```python
from build123d import *

# Parameters (mm, degrees)
EXTRUDE_1_DEPTH     = 5
FILLET_1_R          = 2
SKETCH_2_R          = 1.5
CUT_EXTRUDE_1_DEPTH = 26.495097568
SKETCH_6_R          = 1.5
CUT_EXTRUDE_2_DEPTH = 37.400549446


with BuildPart() as part:
    # 草图1 → 凸台-拉伸1 (new body)
    with BuildSketch(Plane.XY):
        Polygon((9, 20), (9, 12), (-9, 12), (-9, 20), (-15, 20), (-15, -20), (-9, -20), (-9, -12), (9, -12), (9, -20), (15, -20), (15, 20), align=None)
    extrude(amount=EXTRUDE_1_DEPTH)

    # 圆角1
    fillet_1_edges = [part.edges().sort_by_distance(p)[0] for p in [
        (9, -20, 2.5),
        (9, -12, 2.5),
        (-9, -12, 2.5),
        (-9, -20, 2.5),
        (-9, 20, 2.5),
        (-9, 12, 2.5),
        (9, 12, 2.5),
        (9, 20, 2.5),
    ]]
    fillet(fillet_1_edges, radius=FILLET_1_R)

    # 草图2 → 切除-拉伸1 (cut, through all)
    with BuildSketch(Plane.XY.offset(5)):
        with Locations((-5, 5)):
            Circle(SKETCH_2_R)
        with Locations(Location((5, -5, 0), (0, 0, 180))):
            Circle(SKETCH_2_R)
    extrude(amount=-CUT_EXTRUDE_1_DEPTH, mode=Mode.SUBTRACT)

    # 草图6 → 切除-拉伸2 (cut, through all)
    with BuildSketch(Plane(origin=(15, 0, 0), x_dir=(0, 0, -1), z_dir=(1, 0, 0))):
        with Locations(Location((-2.5, 16, 0), (0, 0, 90))):
            Circle(SKETCH_6_R)
        with Locations(Location((-2.5, -16, 0), (0, 0, 90))):
            Circle(SKETCH_6_R)
    extrude(amount=-CUT_EXTRUDE_2_DEPTH, mode=Mode.SUBTRACT)


solid = part.part
```
Here's how the part is built. I have some questions about the finished solid (model axes, mm). A direction names the side the tool comes from. Coordinates: 2 decimals unless noted, no trailing zeros. Order: outer loops, then holes, each group sorted by start corner. A loop starts at its lowest first (then second) coordinate and runs counter-clockwise, first axis right, second up.
Item 1: I need wall thicknesses on probe 1 along X at (y, z) = (15, 4.5); probe 2 along Z at (x, y) = (11.65, 16); probe 3 along X at (y, z) = (-5, 1.4). Which ranges of each line are inside material? Lowest first, please.
Response values:
probe 1: x = -15 to -9, 9 to 15
probe 2: z = 0 to 1, 4 to 5
probe 3: x = -15 to 3.5, 6.5 to 15
Item 2: If we section it at D-D, the plane z = 2.5: Give the number of separate pieces and of enclosed holes in the cut face, then the cut area to 3 significant figures.
Response values:
separate pieces: 5
enclosed holes: 2
area: 826 mm2
Item 3: Thinking about a two-plate mould opening in Y: for faces 1 (the face through (-6.2, 4.1, 2.5)), 2 (the face through (8.43, 12.6, 2.54)), 3 (the face through (12.04, 14.5, 2.57)), 4 (the face through (9, -16, 0.8)), which applies, pulls with the +Y half, pulls with the -Y half, needs draft (parallel to the pull), parting line crosses it, or undercut?
Response values:
face 1: undercut
face 2: pulls with the +Y half
face 3: undercut
face 4: needs draft
Item 4: Which directions (+Z, -Z, +X, -X, +Y, -Y) give clear straight access to the entire face, cutting with the end or side of a thin tool? Please do faces 5 (the face through (9.57, -19.4, 2.54)), 6 (the face through (0, 12, 2)), 7 (the face through (15, 0, 2)).
Response values:
face 5: +Z, -Z, -Y
face 6: +Z, -Z, +Y
face 7: +Z, -Z, +X, +Y, -Y
Item 5: If we section it at C-C, the plane y = -16: List the corners of the cut face in (x, z) for me.
Response values:
outline: (-15, 0) - (-9, 0) - (-9, 1) - (-15, 1) - close; (-15, 4) - (-9, 4) - (-9, 5) - (-15, 5) - close; (9, 0) - (15, 0) - (15, 1) - (9, 1) - close; (9, 4) - (15, 4) - (15, 5) - (9, 5) - close
Item 6: I'm going to push flat-ended pins straight in: pin 1 Ø2 at (x, z) = (-7.5, 1.5) entering from +Y; pin 2 Ø1.8 at (x, y) = (5, -5) entering from +Z. Where does each tip first touch, or does it pass through?
Response values:
pin 1: stops at y = 12.68
pin 2: passes through
Item 7: If we section it at B-B, the plane x = 5: List the corners of the cut face in (y, z) for me, then the cut area to 3 significant figures.
Response values:
outline: (-12, 0) - (-6.5, 0) - (-6.5, 5) - (-12, 5) - close; (-3.5, 0) - (12, 0) - (12, 5) - (-3.5, 5) - close
area: 105 mm2
Item 8: If we section it at A-A, the plane y = -5: List the corners of the cut face in (x, z) for me, then the cut area to 3 significant figures.
Response values:
outline: (-15, 0) - (3.5, 0) - (3.5, 5) - (-15, 5) - close; (6.5, 0) - (15, 0) - (15, 5) - (6.5, 5) - close
area: 135 mm2
